Design review of the part built by this model. Coordinates are the model's own, in mm. A direction names the side the tool comes from. Give positions to 0.01 mm unless a question says otherwise; leave off trailing zeros. Order: outer loops, then holes, each group sorted by start corner. A loop starts at its lowest first (then second) coordinate and runs counter-clockwise, first axis right, second up. Notation, with made-up numbers: (42.5, 62.25) -> (64.5, 62.25) arc R21 ccw to (64.5, 83.25) -> close; hole circle Ø9 at (78, -31.5). An arc over 180 degrees is marked (long way). Return JSON: item names as keys, results as strings.
```python
from build123d import *

# Parameters (mm, degrees)
BASE_EXTRUSION_DEPTH    = 3
ESQUISSE2_R             = 3.5
BOSS_EXTRU_1_DEPTH      = 0.5
CONG_1_R                = 0.5
ENL_V_START             = -1
ENL_V_MAT_EXTRU_1_DEPTH = 1
BOSS_EXTRU_2_START      = 3
ESQUISSE5_R             = 3.5
BOSS_EXTRU_2_DEPTH      = 3
ESQUISSE4_R             = 1.25
ENL_V_MAT_EXTRU_3_DEPTH = 28.354158733
ESQUISSE9_R             = 12
ENL_V_MAT_EXTRU_4_DEPTH = 0.5
BOSS_EXTRU_3_START      = 3
BOSS_EXTRU_3_DEPTH      = 3
ESQUISSE12_R            = 4
ENL_V_MAT_EXTRU_5_DEPTH = 4
ESQUISSE13_R            = 3
ENL_V_MAT_EXTRU_6_DEPTH = 27.949025956


with BuildPart() as part:
    # Esquisse1 → Base-Extrusion (new body)
    with BuildSketch(Plane.XY):
        with BuildLine():
            Line((-8.858707286, 1.588491495), (-7.5, 19.063508327))
            ThreePointArc((-7.5, 19.063508327), (-6.626477999, 24.01688802), (-1.6, 24.2))
            Line((-1.6, 24.2), (1.6, 24.2))
            ThreePointArc((1.6, 24.2), (6.626477999, 24.01688802), (7.5, 19.063508327))
            Line((7.5, 19.063508327), (8.858707286, 1.588491495))
            ThreePointArc((8.858707286, 1.588491495), (0, -9), (-8.858707286, 1.588491495))
        make_face()
    extrude(amount=BASE_EXTRUSION_DEPTH)

    # Esquisse2 → Boss.-Extru.1 (add)
    with BuildSketch(Plane.XY.offset(3)):
        with Locations((4, 21)):
            Circle(ESQUISSE2_R)
        with Locations((-4, 21)):
            Circle(ESQUISSE2_R)
    extrude(amount=BOSS_EXTRU_1_DEPTH)

    # Congé1
    cong_1_edges = [part.edges().sort_by_distance(p)[0] for p in [
        (0.5, 21, 3.5),
        (-7.5, 21, 3.5),
    ]]
    fillet(cong_1_edges, radius=CONG_1_R - 0.0001)  # a hair under: the kernel refuses the full size

    # Esquisse3 → Enlèv. mat.-Extru.1 (cut)
    with BuildSketch(Plane.XY.offset(3).offset(ENL_V_START)):
        with BuildLine():
            Line((-6.543725832, 10.97906245), (-6.097110858, 16.831549851))
            ThreePointArc((-6.097110858, 16.831549851), (-5.866577748, 17.215602456), (-5.420942587, 17.260892865))
            ThreePointArc((-5.420942587, 17.260892865), (-2.327193854, 17.366582931), (-0.235294118, 19.648338201))
            ThreePointArc((-0.235294118, 19.648338201), (0, 19.813859338), (0.235294118, 19.648338201))
            ThreePointArc((0.235294118, 19.648338201), (2.327193854, 17.366582931), (5.420942587, 17.260892865))
            ThreePointArc((5.420942587, 17.260892865), (5.866577748, 17.215602456), (6.097110858, 16.831549851))
            Line((6.097110858, 16.831549851), (6.543725832, 10.97906245))
            ThreePointArc((6.543725832, 10.97906245), (6.315450438, 10.520361161), (5.803368369, 10.503376389))
            ThreePointArc((5.803368369, 10.503376389), (0, 12), (-5.803368369, 10.503376389))
            ThreePointArc((-5.803368369, 10.503376389), (-6.315450438, 10.520361161), (-6.543725832, 10.97906245))
        make_face()
    extrude(amount=ENL_V_MAT_EXTRU_1_DEPTH, mode=Mode.SUBTRACT)

    # Esquisse5 → Boss.-Extru.2 (add)
    with BuildSketch(Plane(origin=(0, 0, 0), x_dir=(-1, 0, 0), z_dir=(0, 0, -1)).offset(BOSS_EXTRU_2_START)):
        with Locations(Location((4, 21, 0), (0, 0, 180))):
            Circle(ESQUISSE5_R)
        with Locations(Location((-4, 21, 0), (0, 0, 180))):
            Circle(ESQUISSE5_R)
    extrude(amount=-BOSS_EXTRU_2_DEPTH)

    # Esquisse4 → Enlèv. mat.-Extru.3 (cut, through all)
    with BuildSketch(Plane.XY.offset(3.5)):
        with Locations((4, 21)):
            Circle(ESQUISSE4_R)
        with Locations((-4, 21)):
            Circle(ESQUISSE4_R)
    extrude(amount=-ENL_V_MAT_EXTRU_3_DEPTH, mode=Mode.SUBTRACT)

    # Esquisse9 → Enlèv. mat.-Extru.4 (cut)
    with BuildSketch(Plane(origin=(0, 0, 0), x_dir=(-1, 0, 0), z_dir=(0, 0, -1))):
        Circle(ESQUISSE9_R)
    extrude(amount=-ENL_V_MAT_EXTRU_4_DEPTH, mode=Mode.SUBTRACT)

    # Esquisse11 → Boss.-Extru.3 (add)
    with BuildSketch(Plane(origin=(0, 0, 0.5), x_dir=(-1, 0, 0), z_dir=(0, 0, -1)).offset(BOSS_EXTRU_3_START)):
        with BuildLine():
            Line((1.5, -5.809475019), (1.5, -8.874119675))
            ThreePointArc((1.5, -8.874119675), (0, -9), (-1.5, -8.874119675))
            Line((-1.5, -8.874119675), (-1.5, -5.809475019))
            ThreePointArc((-1.5, -5.809475019), (0, 6), (1.5, -5.809475019))
        make_face()
    extrude(amount=-BOSS_EXTRU_3_DEPTH)

    # Esquisse12 → Enlèv. mat.-Extru.5 (cut)
    with BuildSketch(Plane.XY.offset(3)):
        Circle(ESQUISSE12_R)
    extrude(amount=-ENL_V_MAT_EXTRU_5_DEPTH, mode=Mode.SUBTRACT)

    # Esquisse13 → Enlèv. mat.-Extru.6 (cut, through all)
    with BuildSketch(Plane.XY.offset(-1)):
        Circle(ESQUISSE13_R)
    extrude(amount=-ENL_V_MAT_EXTRU_6_DEPTH, mode=Mode.SUBTRACT)


solid = part.part
```
Item 1: Mouldability with a two-part tool opening along X and no side actions: class faces 1 (the face through (5, 20, 3.5)), 2 (the face through (1.5, -7, -1)), 3 (the face through (0, 24.2, 1)) as released by +X, released by -X, zero draft, split by the parting line, or undercut.
Result set:
{"face 1": "zero draft", "face 2": "released by +X", "face 3": "undercut"}
Item 2: Add section C-C (y = 21). Give the number of separate pieces and of enclosed holes in the cut face, plus the area to 3 significant figures.
Result set:
{"separate pieces": "3", "enclosed holes": "0", "area": "64.3 mm^2"}
Item 3: Add section B-B (y = 0). Give the boundary of the cut face in (x, z), plus the area to 3 significant figures.
Result set:
{"outline": "(-9, 0.5) -> (-6, 0.5) -> (-6, -2.5) -> (-3, -2.5) -> (-3, -1) -> (-4, -1) -> (-4, 3) -> (-9, 3) -> close; (3, -2.5) -> (6, -2.5) -> (6, 0.5) -> (9, 0.5) -> (9, 3) -> (4, 3) -> (4, -1) -> (3, -1) -> close", "area": "40.0 mm^2"}
Item 4: Add section A-A (z = -1.5). Give the boundary of the cut face in (x, y).
Result set:
{"outline": "circle Ø7 at (-4, 21); (-1.5, -8.87) arc R9 ccw to (1.5, -8.87) -> (1.5, -5.81) arc R6 ccw (long way) to (-1.5, -5.81) -> close; circle Ø7 at (4, 21); hole circle Ø2.5 at (-4, 21); hole circle Ø6 at (0, 0); hole circle Ø2.5 at (4, 21)"}
Item 5: For pin 1 (4 mm diameter, centred on x = 2, y = 1.5, fed in from +Z); pin 2 (9 mm diameter, centred on x = 1, y = -2.5, fed in from -Z); pin 3 (6 mm diameter, centred on x = -6.5, y = 10, fed in from -Z); pin 4 (3 mm diameter, centred on x = 4, y = 21, fed in from -Z), all flat-tipped, find the tip position at first contact; note any pin that passes through.
Result set:
{"pin 1": "stops at z = 3", "pin 2": "stops at z = -2.5", "pin 3": "stops at z = 0", "pin 4": "stops at z = -3"}
Item 6: Wall thickness on L1, parallel to X at y = 18.5, z = -1.25; L2, parallel to X at y = 20, z = 1; L3, parallel to X at y = 19, z = -2.25: over which ranges is each line inside the solid? List them lowest first. Write a range as [from, to].
Result set:
{"L1": "x = [-6.45, -1.55], [1.55, 6.45]", "L2": "x = [-7.87, -4.75], [-3.25, 3.25], [4.75, 7.87]", "L3": "x = [-6.87, -1.13], [1.13, 6.87]"}
Item 7: Add section D-D (z = 1.5). Give the boundary of the cut face in (x, y), plus the area to 3 significant figures.
Result set:
{"outline": "(-8.86, 1.59) arc R9 ccw (long way) to (8.86, 1.59) -> (7.5, 19.06) arc R4 ccw to (1.6, 24.2) -> (-1.6, 24.2) arc R4 ccw to (-7.5, 19.06) -> close; hole circle Ø2.5 at (-4, 21); hole circle Ø8 at (0, 0); hole circle Ø2.5 at (4, 21)", "area": "465 mm^2"}
Item 8: Machinability: for faces 4 (the face through (8.17, 10.45, 1.48)), 5 (the face through (0.1, 6.3, 0.5)), 6 (the face through (-8.19, 10.2, 1.48)), which of the approach directions +Z, -Z, +X, -X, +Y, -Y give a long, thin tool a straight path to every point of the face, cutting with its end or side? Answer none if there is none.
Result set:
{"face 4": "+Z, -Z, +X", "face 5": "-Z", "face 6": "+Z, -Z, -X"}
